Could you check a few things on this model? Use its own coordinates, in mm. Give positions to 0.01 mm unless a question says otherwise; leave off trailing zeros. Loops run counter-clockwise (first coordinate to the right, second up) from the corner with the lowest first, then second, coordinate; pieces in that order, holes last.
1. For P1, Ø4, axis at y = 12, z = -3, coming from the -X side; P2, Ø0.6, axis at x = 1, y = -1, coming from the -Z side; P3, Ø0.6, axis at x = 1, z = -8.5, coming from the -Y side; P4, Ø1, axis at x = 1.5, z = -9.5, coming from the -Y side, each with a flat end and sliding along its axis, tell me the tip position at first contact or that it passes through.
2. Imagine slicing it at A-A (y = -12). List the corners of the cut face in (x, z) for me.
3. Imagine slicing it at C-C (x = 1.3). List the corners of the cut face in (y, z) for me.
4. Imagine slicing it at B-B (z = -10.5). List the corners of the cut face in (x, y) for me, plus the area to 3 significant figures.
5. I need wall thicknesses on line 1 along Y through (x, z) = (1.4, -3); line 2 along Y through (x, z) = (1.55, -12.5); line 3 along Z through (x, y) = (1.9, -17). Which ranges of each line are inside material? Lowest first, please.
6. Thinking about a two-plate mould opening in Z: for faces 1 (the flat face through (1, -20, -4)), 2 (the cylindrical face through (1.014, 13.586, -2.792)), 3 (the cylindrical face through (1, -12, -13)), 4 (the flat face through (1, 0, 0)), which applies, +Z half, -Z half, draft (parallel to the pull), parting line (faces both ways), or undercut?
7. Imagine slicing it at D-D (z = -3). List the corners of the cut face in (x, y) for me.
Autodesk Inventor part; units mm, degrees
ref_plane "YZ Plane" through (0, 0, 0) normal (1, 0, 0) x (0, 1, 0)
ref_plane "XZ Plane" through (0, 0, 0) normal (0, 1, 0) x (-1, 0, 0)
ref_plane "XY Plane" through (0, 0, 0) normal (0, 0, 1) x (1, 0, 0)
sketch "スケッチ1" plane through (0, 0, 0) normal (1, 0, 0) x (0, 1, 0)
  line L0 (20, 0) -> (0, 0)
  line L1 (0, 0) -> (0, -8)
  line L2 (0, -8) -> (20, -8)
  line L3 (20, -8) -> (20, 0)
  circle A0 centre (12, -10.5) radius 2.5 construction
  circle A1 centre (12, -10.5) radius 2.5
  line L4 (13.5, -8.5) -> (10.5, -8.5)
  line L5 (10.5, -8.5) -> (10.5, -8)
  line L6 (10.5, -8) -> (13.5, -8)
  line L7 (13.5, -8) -> (13.5, -8.5)
  line L8 (12, -10.5) -> (12, -8)
  point P0 (13.5, -8)
  point P1 (10.5, -8)
  dimension "d1" = 5
  dimension "d0" = 5
  dimension "d2" = 3
  dimension "d3" = 12
  dimension "d4" = 8
  dimension "d5" = 20
extrude "押し出し1" add sketch "スケッチ1" along normal blind 2
mirror "ミラー1" about plane through (0, 0, 0) normal (0, -1, 0)
sketch "スケッチ2" plane through (2, 0, 0) normal (1, 0, 0) x (0, 0, -1)
  line L0 (8.5, 13.5) -> (8, 13.5)
  line L1 (8, 13.5) -> (8, 20)
  line L2 (8, 20) -> (0, 20)
  line L3 (0, 20) -> (0, -20)
  line L4 (8, -20) -> (0, -20)
  line L5 (8, -13.5) -> (8, -20)
  line L6 (8.5, -13.5) -> (8, -13.5)
  arc A0 (8.5, -13.5) -> (8.5, -10.5) centre (10.5, -12) ccw
  line L7 (8, -10.5) -> (8.5, -10.5)
  line L8 (8, 10.5) -> (8, -10.5)
  line L9 (8, 10.5) -> (8.5, 10.5)
  arc A1 (8.5, 10.5) -> (8.5, 13.5) centre (10.5, 12) ccw
  circle A2 centre (3, 12) radius 1.6
  circle A3 centre (3, -12) radius 1.6
  point P0 (0, 0)
  dimension "d8" = 3.2
  dimension "d17" = 3
extrude "押し出し2" cut sketch "スケッチ2" against normal blind 2 contours A2 | A3
properties part number "cover_setter"
Derived:
1. P1: stops at x = 0
1. P2: stops at z = -8
1. P3: stops at y = -13.83
1. P4: stops at y = -14.45
2. outline: (0, -13) - (2, -13) - (2, -4.6) - (0, -4.6) - close; (0, -1.4) - (2, -1.4) - (2, 0) - (0, 0) - close
3. outline: (-20, -8) - (-13.5, -8) - (-13.5, -8.5) arc R2.5 ccw (long way) to (-10.5, -8.5) - (-10.5, -8) - (10.5, -8) - (10.5, -8.5) arc R2.5 ccw (long way) to (13.5, -8.5) - (13.5, -8) - (20, -8) - (20, 0) - (-20, 0) - close; hole circle Ø3.2 at (-12, -3); hole circle Ø3.2 at (12, -3)
4. outline: (0, -14.5) - (2, -14.5) - (2, -9.5) - (0, -9.5) - close; (0, 9.5) - (2, 9.5) - (2, 14.5) - (0, 14.5) - close
4. area: 20.0 mm2
5. line 1: y = -20 to -13.6, -10.4 to 10.4, 13.6 to 20
5. line 2: y = -13.5 to -10.5, 10.5 to 13.5
5. line 3: z = -8 to 0
6. face 1: draft
6. face 2: undercut
6. face 3: undercut
6. face 4: +Z half
7. outline: (0, -20) - (2, -20) - (2, -13.6) - (0, -13.6) - close; (0, -10.4) - (2, -10.4) - (2, 10.4) - (0, 10.4) - close; (0, 13.6) - (2, 13.6) - (2, 20) - (0, 20) - close
